Study the drawing (mm; zero at the part's minimum x, y, z) and answer. Coordinates: 2 decimals unless noted, no trailing zeros. Order: outer loops, then holes, each group sorted by start corner. A loop starts at its lowest first (then second) coordinate and runs counter-clockwise, first axis right, second up.
1. The part is cut by section A-A, the plane x = 209.55. Give the vertices of the cut face in (y, z) (1 decimal).
2. Flat-ended cylindrical pins translate along their axes: pin 1 Ø1.9 at (x, z) = (90, 2) entering from -Y; pin 2 Ø1 at (x, y) = (83, 72) entering from -Z; pin 3 Ø1.9 at (y, z) = (6, 4) entering from +X. Find the tip coordinate at first contact, or state that the pin passes through.
3. Find the intervals of material crossed by probe 1 along X at (y, z) = (292.1, 1.5) (1 decimal); probe 2 along Y at (x, z) = (209.55, 3.75); probe 3 along Y at (x, z) = (32, 5.5), in increasing order.
4. The part is cut by section B-B, the plane z = 1.5. Count the separate pieces of the cut face and the enclosed holes in it, then the cut area to 3 significant figures.
5. The part is cut by section C-C, the plane x = 128. Give the vertices of the cut face in (y, z) (1 decimal), then the cut area to 3 significant figures.
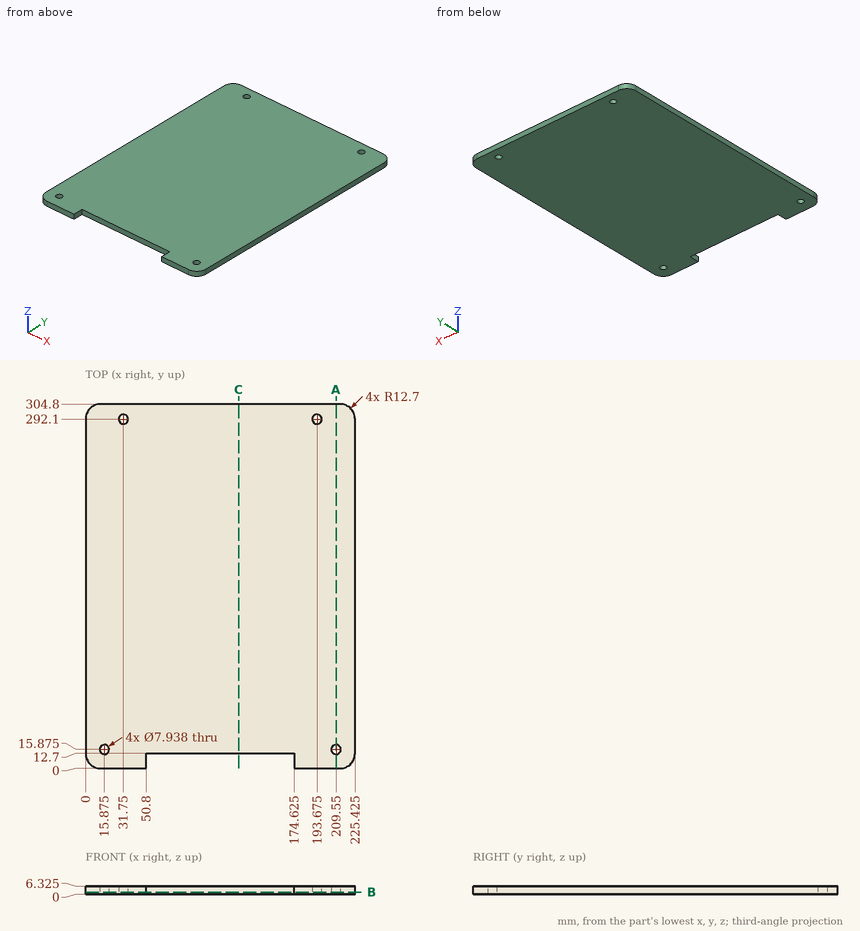
Geometry says:
1. outline: (0, 0) - (11.9, 0) - (11.9, 6.3) - (0, 6.3) - close; (19.8, 0) - (304.8, 0) - (304.8, 6.3) - (19.8, 6.3) - close
2. pin 1: stops at y = 12.7
2. pin 2: stops at z = 0
2. pin 3: stops at x = 224.05
3. probe 1: x = 0 to 27.8, 35.7 to 189.7, 197.6 to 225.4
3. probe 2: y = 0 to 11.91, 19.84 to 304.8
3. probe 3: y = 0 to 288.14, 296.06 to 304.8
4. separate pieces: 1
4. enclosed holes: 4
4. area: 66,800 mm2
5. outline: (12.7, 0) - (304.8, 0) - (304.8, 6.3) - (12.7, 6.3) - close
5. area: 1,850 mm2
